Answer from the drawing. Dimensions are ordinates in mm from the lowest x, y and z of the part. A direction names the side the tool comes from. Give positions to 0.01 mm unless a question says otherwise; leave off trailing zeros. Write each loop counter-clockwise with the first axis right and the second up, starting at its lowest first coordinate (ties: lowest second). Pieces come first, ordered by that corner, then holes. Notation, with made-up numbers: (73, 48) - (92, 48) arc R19 cw to (92, 71) - close; hole circle Ø3 at (40.25, 33.25). An arc over 180 degrees is marked (long way). Answer as a JSON object with one key per item and string values. Group by question number.
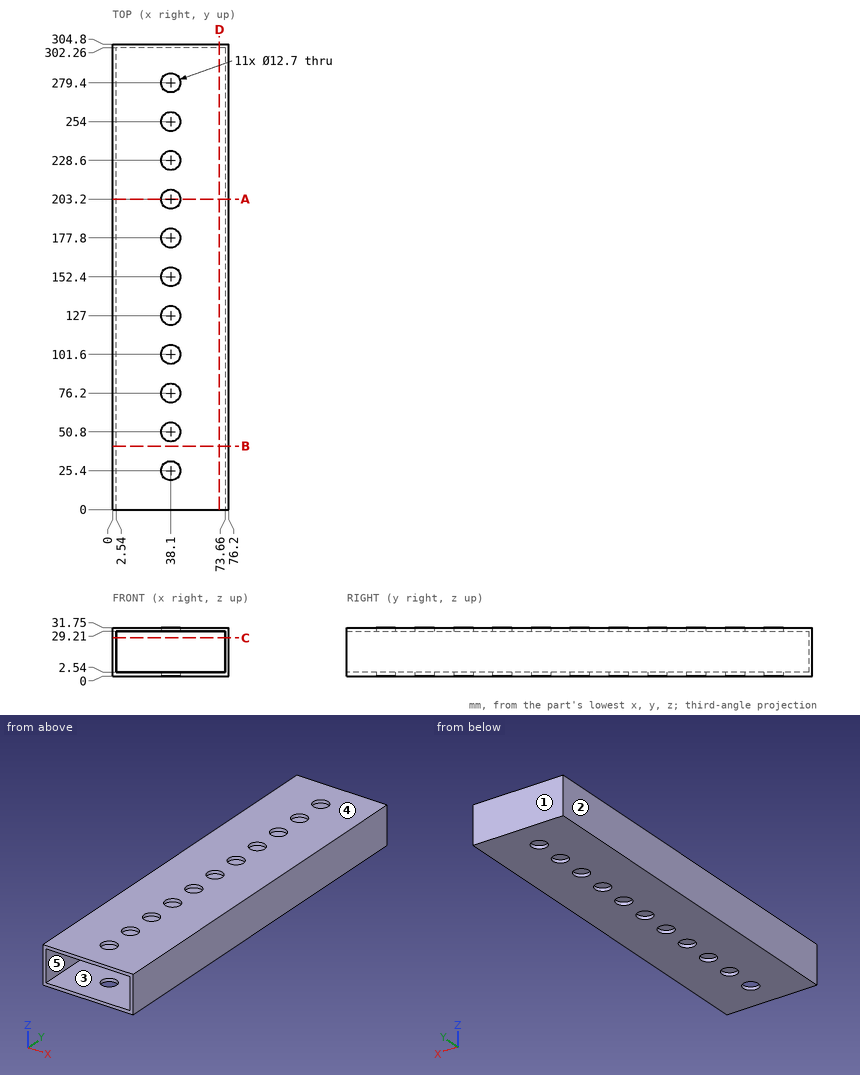
1) Find section D-D, the plane x = 70. Write down the section's boundary in (y, z), and give its area (3 significant figures).
2) Find the intervals of material crossed by line 1 (Z direction, x = 61, y = 111); line 2 (X direction, y = 242.5, z = 6.5); line 3 (X direction, y = 50, z = 31), in increasing order. Write a range as [from, to].
3) Flat-ended cylindrical pins translate along their axes: pin 1 Ø2 at (x, z) = (43, 19) entering from -Y; pin 2 Ø11.5 at (x, y) = (38.1, 50.8) entering from +Z; pin 3 Ø14.5 at (x, y) = (38.1, 76.2) entering from -Z. Find the tip coordinate at first contact, or state that the pin passes through.
4) For a pull along X with two mould halves and no side action, classify the marked faces 1, 2 and 3 as released by +X, released by -X, zero draft, split by the parting line, or undercut.
5) Find section B-B, the plane y = 41.5. Write down the section's boundary in (x, z).
6) Find section C-C, the plane z = 25. Write down the section's boundary in (x, y), and give its area (3 significant figures).
7) Which of the six approach directions +Z, -Z, +X, -X, +Y, -Y give full straight-line access (tool end or side, diameter ignored) to the marked faces 4 and 5?
8) Find section A-A, the plane y = 203.2. Write down the section's boundary in (x, z), and give its area (3 significant figures).
Values follow:
{
 "1": {"outline": "(0, 0) - (304.8, 0) - (304.8, 31.75) - (0, 31.75) - (0, 29.21) - (302.26, 29.21) - (302.26, 2.54) - (0, 2.54) - close", "area": "1,620 mm2"},
 "2": {"line 1": "z = [0, 2.54], [29.21, 31.75]", "line 2": "x = [0, 2.54], [73.66, 76.2]", "line 3": "x = [0, 31.8], [44.4, 76.2]"},
 "3": {"pin 1": "stops at y = 302.26", "pin 2": "passes through", "pin 3": "stops at z = 0"},
 "4": {"face 1": "zero draft", "face 2": "released by -X", "face 3": "undercut"},
 "5": {"outline": "(0, 0) - (76.2, 0) - (76.2, 31.75) - (0, 31.75) - close; hole (2.54, 2.54) - (73.66, 2.54) - (73.66, 29.21) - (2.54, 29.21) - close"},
 "6": {"outline": "(0, 0) - (2.54, 0) - (2.54, 302.26) - (73.66, 302.26) - (73.66, 0) - (76.2, 0) - (76.2, 304.8) - (0, 304.8) - close", "area": "1,730 mm2"},
 "7": {"face 4": "+Z, +X, -X, +Y, -Y", "face 5": "-Y"},
 "8": {"outline": "(0, 0) - (31.75, 0) - (31.75, 2.54) - (2.54, 2.54) - (2.54, 29.21) - (31.75, 29.21) - (31.75, 31.75) - (0, 31.75) - close; (44.45, 0) - (76.2, 0) - (76.2, 31.75) - (44.45, 31.75) - (44.45, 29.21) - (73.66, 29.21) - (73.66, 2.54) - (44.45, 2.54) - close", "area": "458 mm2"}
}
